Input: part model. Units: mm. Frame: model coordinates. Give positions to 0.01 mm unless a question says otherwise; leave off trailing zeros. Loops run counter-clockwise (first coordinate to the right, second up) from the corner with the lowest first, then second, coordinate; pieces in that order, holes last. Notation, with made-up numbers: (10.5, 71.25) -> (60.5, 71.25) arc R16 ccw to (60.5, 88.25) -> close; hole circle Ø3 at (24.5, 4.5). An arc over 180 degrees is marked (long way). One line per question, with ' | ' between items.
from build123d import *

# Parameters (mm, degrees)
SKETCH1_W                   = 12
SKETCH1_H                   = 45
BOSS_EXTRUDE1_DEPTH         = 85
TAP_DRILL_FOR_M5X0_8_TAP1_D = 4.2
FILLET1_R                   = 2


with BuildPart() as part:
    # Sketch1 → Boss-Extrude1 (new body)
    with BuildSketch(Plane(origin=(0, 0, 0), x_dir=(1, 0, 0), z_dir=(0, 1, 0))):
        with Locations((0, -7.5)):
            Rectangle(SKETCH1_W, SKETCH1_H)
    extrude(amount=-BOSS_EXTRUDE1_DEPTH)

    # Tap Drill for M5x0.8 Tap1 (through all)
    with Locations(Plane(origin=(0, 0, -10), x_dir=(0, 0, 1), z_dir=(0, 1, 0))):
        with Locations((0, 0), (20, 0), (35, 0)):
            Hole(TAP_DRILL_FOR_M5X0_8_TAP1_D / 2)

    # Fillet1
    fillet1_edges = [part.edges().sort_by_distance(p)[0] for p in [
        (6, -42.5, 30),
        (-6, -42.5, 30),
        (-6, -42.5, -15),
        (6, -42.5, -15),
    ]]
    fillet(fillet1_edges, radius=FILLET1_R)


solid = part.part
1. Pin query (flat end, axial travel): P1, Ø4, axis at x = 0, z = 10, coming from the -Y side. Return the tip coordinate at first contact, or that it passes through.
Determined:
P1: passes through
2. Ray query, line 1 along X through (y, z) = (-35, 25); line 2 along Z through (x, y) = (0.75, -38.5); line 3 along Z through (x, y) = (1.75, -15.5). Return the intervals inside material, ascending. Write a range as from..to.
Determined:
line 1: x = -6..-2.1, 2.1..6 | line 2: z = -15..-11.96, -8.04..8.04, 11.96..23.04, 26.96..30 | line 3: z = -15..-11.16, -8.84..8.84, 11.16..23.84, 26.16..30
3. Section query A-A (z = -10). Output: boundary loops of the cut face in (x, y), then the cut area to 3 significant figures.
Determined:
outline: (-6, -85) -> (-2.1, -85) -> (-2.1, 0) -> (-6, 0) -> close; (2.1, -85) -> (6, -85) -> (6, 0) -> (2.1, 0) -> close | area: 663 mm2
4. Pull-direction query (Z, two-part tool) for faces 1 (the cylindrical face through (5.4, -43.1, -14.43)), 2 (the cylindrical face through (0.09, -43.1, 12.1)), 3 (the flat face through (0, -85, 7)); classes: pulls with the +Z half, pulls with the -Z half, needs draft (parallel to the pull), parting line crosses it, or undercut.
Determined:
face 1: pulls with the -Z half | face 2: undercut | face 3: needs draft
5. Section query C-C (y = -61). Output: boundary loops of the cut face in (x, z), then the cut area to 3 significant figures.
Determined:
outline: (-6, -13) arc R2 ccw to (-4, -15) -> (4, -15) arc R2 ccw to (6, -13) -> (6, 28) arc R2 ccw to (4, 30) -> (-4, 30) arc R2 ccw to (-6, 28) -> close; hole circle Ø4.2 at (0, -10); hole circle Ø4.2 at (0, 10); hole circle Ø4.2 at (0, 25) | area: 495 mm2
6. Section query B-B (x = 0). Output: boundary loops of the cut face in (y, z).
Determined:
outline: (-85, -15) -> (0, -15) -> (0, -12.1) -> (-85, -12.1) -> close; (-85, -7.9) -> (0, -7.9) -> (0, 7.9) -> (-85, 7.9) -> close; (-85, 12.1) -> (0, 12.1) -> (0, 22.9) -> (-85, 22.9) -> close; (-85, 27.1) -> (0, 27.1) -> (0, 30) -> (-85, 30) -> close
